```python
from build123d import *

# Parameters (mm, degrees)
F0_W     = 20
F0_H     = 31.5
F0_R     = 3
F1_DEPTH = 16
F2_DEPTH = 5
F3_W     = 79.5
F3_H     = 29.5
F4_DEPTH = 1
F5_R     = 1
F6_DEPTH = 17
F7_R     = 3


# Not quite as in the source:
# - a feature names something its author has since deleted; it is built from what else it names


with BuildPart() as f1:
    # F0 (on Top) → F1 (new body)
    with BuildSketch(Plane.XY):
        Polygon((-35.75, -15.75), (-35.75, 15.75), (40.25, 15.75), (45.75, 15.75), (65.75, 15.75), (65.75, 23.75), (-65.75, 23.75), (-65.75, -23.75), (65.75, -23.75), (65.75, -15.75), (45.75, -15.75), (20.25, -15.75), align=None)
        Polygon((-51.7662831426, -2.3), (-55.75, -4.6), (-59.7337168574, -2.3), (-59.7337168574, 2.3), (-55.75, 4.6), (-51.7662831426, 2.3), align=None, mode=Mode.SUBTRACT)
        with Locations((55.75, 0)):
            Rectangle(F0_W, F0_H)
        Polygon((59.7337168574, -2.3), (55.75, -4.6), (51.7662831426, -2.3), (51.7662831426, 2.3), (55.75, 4.6), (59.7337168574, 2.3), align=None, mode=Mode.SUBTRACT)
        Polygon((-59.7337168574, -2.3), (-55.75, -4.6), (-51.7662831426, -2.3), (-51.7662831426, 2.3), (-55.75, 4.6), (-59.7337168574, 2.3), align=None)
        with Locations((-55.75, 0)):
            Circle(F0_R, mode=Mode.SUBTRACT)
        Polygon((51.7662831426, -2.3), (55.75, -4.6), (59.7337168574, -2.3), (59.7337168574, 2.3), (55.75, 4.6), (51.7662831426, 2.3), align=None)
        with Locations((55.75, 0)):
            Circle(F0_R, mode=Mode.SUBTRACT)
    extrude(amount=F1_DEPTH)

    # F0 (on Top) → F2 (join)
    with BuildSketch(Plane.XY):
        Polygon((-35.75, -15.75), (-35.75, 15.75), (40.25, 15.75), (45.75, 15.75), (65.75, 15.75), (65.75, 23.75), (-65.75, 23.75), (-65.75, -23.75), (65.75, -23.75), (65.75, -15.75), (45.75, -15.75), (20.25, -15.75), align=None)
        Polygon((-51.7662831426, -2.3), (-55.75, -4.6), (-59.7337168574, -2.3), (-59.7337168574, 2.3), (-55.75, 4.6), (-51.7662831426, 2.3), align=None, mode=Mode.SUBTRACT)
        with Locations((55.75, 0)):
            Rectangle(F0_W, F0_H)
        Polygon((59.7337168574, -2.3), (55.75, -4.6), (51.7662831426, -2.3), (51.7662831426, 2.3), (55.75, 4.6), (59.7337168574, 2.3), align=None, mode=Mode.SUBTRACT)
        Polygon((40.25, 15.75), (-35.75, 15.75), (-35.75, -15.75), (20.25, -15.75), (45.75, -15.75), (45.75, 15.75), align=None)
    extrude(amount=-F2_DEPTH)

    # F3 (on face) → F4 (cut)
    with BuildSketch(Plane.XY):
        Polygon((45.75, 15.75), (40.25, 15.75), (-35.75, 15.75), (-35.75, -15.75), (20.25, -15.75), (45.75, -15.75), align=None)
        with Locations((5, 0)):
            Rectangle(F3_W, F3_H, mode=Mode.SUBTRACT)
    extrude(amount=-F4_DEPTH, mode=Mode.SUBTRACT)

    # F5 (on face) → F6 (cut, through all)
    with BuildSketch(Plane.XY.offset(16)):
        with Locations((45.75, 15.75)):
            Circle(F5_R)
        with Locations((45.75, -15.75)):
            Circle(F5_R)
        with Locations((-35.75, -15.75)):
            Circle(F5_R)
        with Locations((-35.75, 15.75)):
            Circle(F5_R)
    extrude(amount=-F6_DEPTH, mode=Mode.SUBTRACT)

    # F7
    f7_edges = [f1.edges().sort_by_distance(p)[0] for p in [
        (65.75, 23.75, 5.5),
        (65.75, 0, 16),
        (0, 23.75, 16),
        (0, -23.75, 16),
        (65.75, -23.75, 5.5),
        (-65.75, -23.75, 5.5),
        (-65.75, 23.75, 5.5),
        (-65.75, 0, 16),
    ]]
    fillet(f7_edges, radius=F7_R)


solid = f1.part
```
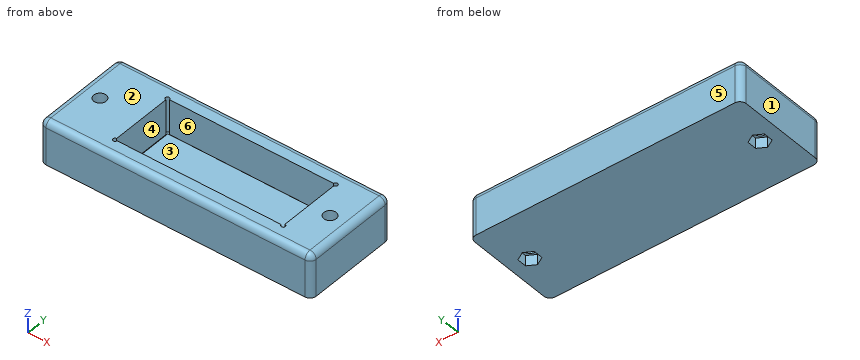
Geometry check sheet. Reference: the model listing, model coordinates, mm. Face numbers are marked on the shaded views. A direction names the side the tool comes from. Give positions to 0.01 mm unless a question says otherwise; leave off trailing zeros. Write each loop counter-clockwise with the first axis right and the second up, starting at its lowest first coordinate (ties: lowest second). Pieces come first, ordered by that corner, then holes. Notation, with made-up numbers: (-35.75, 36) -> (-24.75, 36) arc R24 cw to (-24.75, 66) -> close; hole circle Ø5 at (14, 48.5). An arc over 180 degrees is marked (long way). Use one line per item in the form item = value.
Item 1: Depth check by flat-ended pin: pin 1 Ø3 at (x, y) = (17.5, -8.5) entering from +Z. Enter the tip coordinate at first touch or a pass-through.
Results list:
pin_1 = 0
Item 2: Scan lines: line 1 (Y direction, x = 31, z = 11.75); line 2 (Y direction, x = 55.75, z = 5.5); line 3 (X direction, y = -2, z = 14). Record each from-to range of solid material in increasing order.
Results list:
line_1 = -23.75 to -15.75, 15.75 to 23.75
line_2 = -23.75 to -3, 3 to 23.75
line_3 = -65.58 to -57.99, -53.51 to -35.75, 45.75 to 53.51, 57.99 to 65.58
Item 3: Mould release check, pull along X, two halves, no side actions. Record for the marked faces 1, 2, 3 and 4: released by +X, released by -X, zero draft, split by the parting line, or undercut.
Results list:
face_1 = released by -X
face_2 = zero draft
face_3 = undercut
face_4 = undercut
Item 4: Sectioned sample at A-A on z = 10.75. Enter the section's corners in (x, y).
Results list:
outline = (-65.75, -20.75) arc R3 ccw to (-62.75, -23.75) -> (62.75, -23.75) arc R3 ccw to (65.75, -20.75) -> (65.75, 20.75) arc R3 ccw to (62.75, 23.75) -> (-62.75, 23.75) arc R3 ccw to (-65.75, 20.75) -> close; hole circle Ø6 at (-55.75, 0); hole (-35.75, -14.75) arc R1 ccw (long way) to (-34.75, -15.75) -> (44.75, -15.75) arc R1 ccw (long way) to (45.75, -14.75) -> (45.75, 14.75) arc R1 ccw (long way) to (44.75, 15.75) -> (-34.75, 15.75) arc R1 ccw (long way) to (-35.75, 14.75) -> close; hole circle Ø6 at (55.75, 0)
Item 5: Sectioned sample at B-B on y = -7. Enter the section's corners in (x, z), plus the area to 3 significant figures.
Results list:
outline = (-65.75, -5) -> (65.75, -5) -> (65.75, 13) arc R3 ccw to (62.75, 16) -> (45.75, 16) -> (45.75, -1) -> (44.75, -1) -> (44.75, 0) -> (-34.75, 0) -> (-34.75, -1) -> (-35.75, -1) -> (-35.75, 16) -> (-62.75, 16) arc R3 ccw to (-65.75, 13) -> close
area = 1,450 mm2
Item 6: Access from +Z, -Z, +X, -X, +Y, -Y to the whole of each face (thin tool, end or side, straight path). Record for the marked faces 5 and 6.
Results list:
face_5 = +Z, -Z, +X, -X, +Y
face_6 = +Z
Item 7: Sectioned sample at C-C on x = 17. Enter the section's corners in (y, z), plus the area to 3 significant figures.
Results list:
outline = (-23.75, -5) -> (23.75, -5) -> (23.75, 13) arc R3 ccw to (20.75, 16) -> (15.75, 16) -> (15.75, -1) -> (14.75, -1) -> (14.75, 0) -> (-14.75, 0) -> (-14.75, -1) -> (-15.75, -1) -> (-15.75, 16) -> (-20.75, 16) arc R3 ccw to (-23.75, 13) -> close
area = 488 mm2
